For this review, use the dimensioned drawing (mm, ordinates from the lowest corner) and the shaded views. A direction names the side the tool comes from. Coordinates: 2 decimals unless noted, no trailing zeros. Write each loop counter-clockwise with the first axis right and the second up, starting at its lowest first coordinate (ties: lowest second). Pieces come first, ordered by that corner, then holes. Notation, with made-up numbers: M 46.25,74.25 L 68.25,74.25 A9 ccw 68.25,88.25 Z; hole C -24,38.25 d4. An arc over 180 degrees is marked long. One line per question, with ' | ' between items.
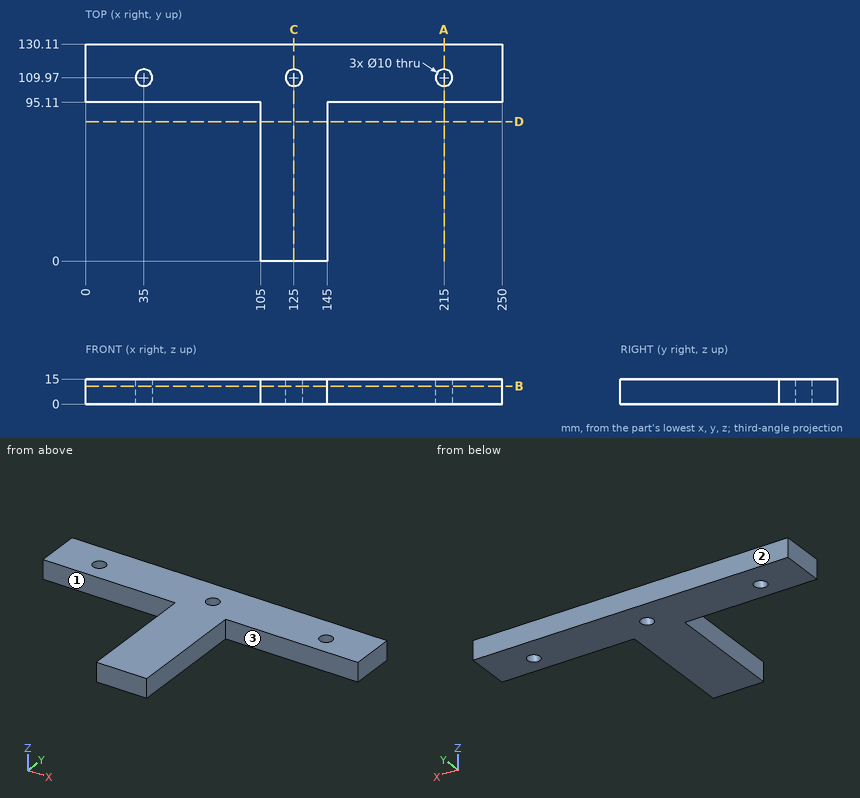
1. Take a section at D-D (y = 83.5). Write out the cut boundary in (x, z), then the cut area to 3 significant figures.
Answer sheet:
outline: M 105,0 L 145,0 L 145,15 L 105,15 Z | area: 600 mm^2
2. Insertion check: pin 1 Ø4.5 at (x, z) = (218.5, 6.5) entering from -Y; pin 2 Ø2 at (y, z) = (17.5, 4) entering from -X; pin 3 Ø11.5 at (x, y) = (125, 109.97) entering from +Z. Each pin has a flat end and moves straight along its axis. Give the tip position at first contact, or say it passes through.
Answer sheet:
pin 1: y = 95.11 | pin 2: x = 105 | pin 3: z = 15
3. Take a section at B-B (z = 10.75). Write out the cut boundary in (x, y).
Answer sheet:
outline: M 0,95.11 L 105,95.11 L 105,0 L 145,0 L 145,95.11 L 250,95.11 L 250,130.11 L 0,130.11 Z; hole C 35,109.97 d10; hole C 125,109.97 d10; hole C 215,109.97 d10
4. Take a section at C-C (x = 125). Write out the cut boundary in (y, z).
Answer sheet:
outline: M 0,0 L 104.97,0 L 104.97,15 L 0,15 Z; M 114.97,0 L 130.11,0 L 130.11,15 L 114.97,15 Z
5. To check wall thickness, follow line 1 along Y through (x, z) = (35.5, 14) (3 decimals); line 2 along Y through (x, z) = (215, 11); line 3 along X through (y, z) = (111, 10.5). State the ranges of each line that lie inside material, in increasing order. Write a range as [from, to].
Answer sheet:
line 1: [95.11, 104.995], [114.945, 130.11] | line 2: [95.11, 104.97], [114.97, 130.11] | line 3: [0, 30.11], [39.89, 120.11], [129.89, 210.11], [219.89, 250]
6. Tool access review of the marked faces 1, 2 and 3: name each direction out of +Z, -Z, +X, -X, +Y, -Y from which nothing blocks a thin tool from reaching the whole face with its end or side.
Answer sheet:
face 1: +Z, -Z, -X, -Y | face 2: +Z, -Z, +X, -X, +Y | face 3: +Z, -Z, +X, -Y
7. Take a section at A-A (x = 215). Write out the cut boundary in (y, z).
Answer sheet:
outline: M 95.11,0 L 104.97,0 L 104.97,15 L 95.11,15 Z; M 114.97,0 L 130.11,0 L 130.11,15 L 114.97,15 Z
